Can you work these out from the model? Positions are in its coordinate system, mm. Face numbers are marked on the shaded views. A direction names the side the tool comes from. Round coordinates to 2 decimals unless told otherwise and drop trailing zeros. Order: outer loops, then holes, each group sorted by start corner. A loop starts at its lowest first (then second) coordinate and runs counter-clockwise, first axis right, second up. Notation, with made-up numbers: (55, -25) -> (71, -25) arc R29 cw to (71, 2) -> close; hole circle Ø1 at (71, -14.5). An arc over 180 degrees is marked (long way). Use a Markdown table: item, result. Add a question column.
Q1. We'd pull the mould along Z, two halves only. Please class the marked faces 1, 2, 3 and 4: +Z half, -Z half, draft (parallel to the pull), parting line (faces both ways), or undercut.
Q2. I'm going to push flat-ended pins straight in: pin 1 Ø4 at (x, z) = (-57, -4.5) entering from +Y; pin 2 Ø3 at (x, z) = (-9.5, 3) entering from -Y; pin 3 Ø12 at (y, z) = (5.5, -8.5) entering from +X. Where does each tip first touch, or does it pass through?
Q3. I need wall thicknesses on line 1 along X through (y, z) = (-2, -5.5); line 2 along X through (y, z) = (-1.75, 5.5); line 3 along Y through (x, z) = (-59.5, -5). Which ranges of each line are inside material? Lowest first, please. Write a range as [from, to].
Q4. For the marked faces 5, 6 and 7, which set-ups out of +Z, -Z, +X, -X, +Y, -Y let a thin tool reach every point of the face, with its end or its side?
Q5. If we section it at A-A on x = -49: List the corners of the cut face in (y, z) for me, plus the area to 3 significant figures.
Q6. If we section it at B-B on x = -32: List the corners of the cut face in (y, z) for me.
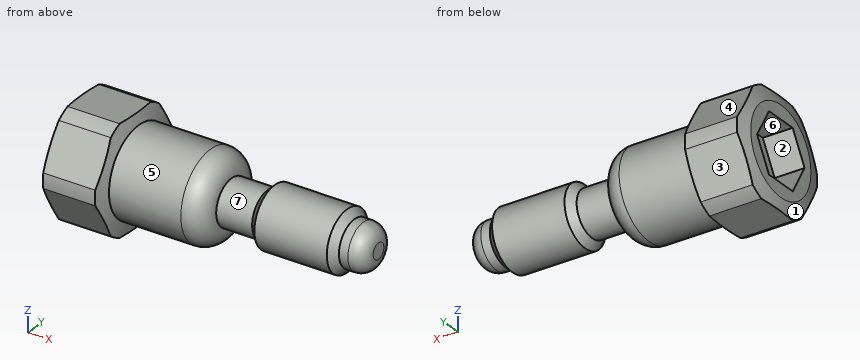
```python
from build123d import *

# Parameters (mm, degrees)
F3_DEPTH = 6.35
F4_R     = 15.610651
F5_DEPTH = 25.4


with BuildPart() as f1:
    # F0 (on Front) → F1 (revolve)
    with BuildSketch(Plane.XZ):
        with BuildLine():
            Line((-63.5, 0), (0, 0))
            Line((0, 0), (0, 1.651))
            ThreePointArc((0, 1.651), (-0.929936, 3.896064), (-3.175, 4.826))
            Line((-3.175, 4.826), (-5.08, 4.826))
            Line((-5.08, 4.826), (-6.604, 6.35))
            Line((-6.604, 6.35), (-21.971, 6.35))
            Line((-21.971, 6.35), (-23.495, 4.826))
            Line((-23.495, 4.826), (-31.115, 4.826))
            ThreePointArc((-31.115, 4.826), (-32.41691, 7.96909), (-35.56, 9.271))
            Line((-35.56, 9.271), (-50.8, 9.271))
            Line((-50.8, 9.271), (-51.637127, 12.3952))
            Line((-51.637127, 12.3952), (-62.662873, 12.3952))
            Line((-62.662873, 12.3952), (-63.5, 9.271))
            Line((-63.5, 9.271), (-63.5, 0))
        make_face()
    revolve(axis=Axis((-31.75, 0, 0), (-1, 0, 0)))

    # F2 (on face) → F3 (cut)
    with BuildSketch(Plane(origin=(-63.5, 0, 0), x_dir=(0, -1, 0), z_dir=(-1, 0, 0))):
        Polygon((3.666174, 6.35), (-3.666174, 6.35), (-7.332348, 0), (-3.666174, -6.35), (3.666174, -6.35), (7.332348, 0), align=None)
    extrude(amount=-F3_DEPTH, mode=Mode.SUBTRACT)

    # F4 (on face) → F5 (cut)
    with BuildSketch(Plane(origin=(-63.5, 0, 0), x_dir=(0, -1, 0), z_dir=(-1, 0, 0))):
        Circle(F4_R)
        Polygon((-13.198227, 0), (-6.599114, 11.43), (6.599114, 11.43), (13.198227, 0), (6.599114, -11.43), (-6.599114, -11.43), align=None, mode=Mode.SUBTRACT)
    extrude(amount=-F5_DEPTH, mode=Mode.SUBTRACT)


solid = f1.part
```
Answer below:
| question | item | result |
|---|---|---|
| 1 | face 1 | parting line |
| 1 | face 2 | undercut |
| 1 | face 3 | -Z half |
| 1 | face 4 | +Z half |
| 2 | pin 1 | y = 11.75 |
| 2 | pin 2 | y = -6.17 |
| 2 | pin 3 | x = -1.18 |
| 3 | line 1 | [-57.15, -31.24], [-22.47, -6.11] |
| 3 | line 2 | [-57.15, -31.22], [-22.55, -6.03] |
| 3 | line 3 | [-10.31, -4.45], [4.45, 10.31] |
| 4 | face 5 | +X |
| 4 | face 6 | -X |
| 4 | face 7 | none |
| 5 | outline | circle Ø18.54 at (0, 0) |
| 5 | area | 270 mm² |
| 6 | outline | circle Ø14.98 at (0, 0) |
